Verification items for the finished model (mm, model axes). Face numbers are marked on the shaded views. A direction names the side the tool comes from. Give positions to 0.01 mm unless a question says otherwise; leave off trailing zeros. Order: outer loops, then holes, each group sorted by start corner. A loop starts at its lowest first (then second) coordinate and runs counter-clockwise, first axis right, second up.
(1) Sectioned sample at A-A on y = 0. Record the cut outline in (x, z), plus the area to 3 significant figures.
(2) Sectioned sample at D-D on z = 18.75. Record the cut outline in (x, y).
(3) Sectioned sample at C-C on y = 11.75. Record the cut outline in (x, z).
(4) Mould release check, pull along Z, two halves, no side actions. Record for the marked faces 1, 2 and 3: pulls with the +Z half, pulls with the -Z half, needs draft (parallel to the pull), parting line crosses it, or undercut.
(5) Sectioned sample at B-B on x = -59. Record the cut outline in (y, z).
(6) Access from +Z, -Z, +X, -X, +Y, -Y to the whole of each face (thin tool, end or side, straight path). Record for the marked faces 4, 5 and 6.
(7) Scan lines: L1, parallel to X at y = -1.5, z = 6.25; L2, parallel to Z at x = -62, y = 7.5; L3, parallel to Z at x = -62.5, y = 5.25. Record each from-to range of solid material in increasing order.
(8) Gauge pin test, flat ends, axial feed: pin 1 (2 mm diameter, centred on y = 3.5, z = 6.5, fed in from -X); pin 2 (3 mm diameter, centred on x = -62.5, y = -1.5, fed in from +Z); pin 3 (3 mm diameter, centred on x = -55, y = 14.89, fed in from +Z); pin 4 (1.5 mm diameter, centred on y = 11, z = 17, fed in from +X). Record the tip position at first contact, or that the pin passes through.
```python
from build123d import *

# Parameters (mm, degrees)
BOSS_EXTRUDE1_DEPTH     = 20
SKETCH2_R               = 2.5
CUT_EXTRUDE1_DEPTH      = 71.632853546
BOSS_EXTRUDE4_DEPTH     = 10
CUT_EXTRUDE2_DEPTH      = 80.703956491
CUT_EXTRUDE2_DEPTH_BACK = 80.703956491
SKETCH6_W               = 5.08
SKETCH6_H               = 17.7
SKETCH7_R               = 0.889
CUT_EXTRUDE3_DEPTH      = 73.716888558
CUT_EXTRUDE4_DEPTH      = 73.716888558
CUT_EXTRUDE4_DEPTH_BACK = 73.716888558
SKETCH8_W               = 40
SKETCH8_H               = 4.572
SKETCH8_W_2             = 60
SKETCH8_H_2             = 5
SKETCH4_R               = 7.5
SKETCH4_R_2             = 2.5
BOSS_EXTRUDE3_DEPTH     = 3
CHAMFER1_SIZE           = 5
BOSS_EXTRUDE2_START     = 3
SKETCH3_R               = 5
SKETCH3_R_2             = 2.5
BOSS_EXTRUDE2_DEPTH     = 3
CHAMFER2_SIZE           = 3


with BuildPart() as part:
    # Sketch1 → Boss-Extrude1 (new body)
    with BuildSketch(Plane.XY):
        with BuildLine():
            Line((-60.35, 6.991244524), (-0.5, 9.987492178))
            ThreePointArc((-0.5, 9.987492178), (10, 0), (-0.5, -9.987492178))
            Line((-0.5, -9.987492178), (-60.35, -6.991244524))
            ThreePointArc((-60.35, -6.991244524), (-67, 0), (-60.35, 6.991244524))
        make_face()
    extrude(amount=BOSS_EXTRUDE1_DEPTH)

    # Sketch2 → Cut-Extrude1 (cut, through all)
    with BuildSketch(Plane.XY.offset(20)):
        with Locations((-60, 0)):
            Circle(SKETCH2_R)
        Circle(SKETCH2_R)
    extrude(amount=-CUT_EXTRUDE1_DEPTH, mode=Mode.SUBTRACT)

    # Sketch5 → Boss-Extrude4 (add)
    with BuildSketch(Plane.XY):
        with BuildLine():
            Line((-60.35, 6.991244524), (-45.63025704, 7.728153385))
            Line((-45.63025704, 7.728153385), (-50.477534128, 17.202429338))
            ThreePointArc((-50.477534128, 17.202429338), (-55.254, 19.962268451), (-59.730944827, 16.739179378))
            Line((-59.730944827, 16.739179378), (-63.60774296, 6.828153385))
            Line((-63.60774296, 6.828153385), (-64.043561758, 5.713983576))
            ThreePointArc((-64.043561758, 5.713983576), (-62.287727062, 6.615610697), (-60.35, 6.991244524))
        make_face()
    extrude(amount=BOSS_EXTRUDE4_DEPTH)

    # Sketch6 → Cut-Extrude2 (cut, two sides: drawn at the far end of the back side and taken through both)
    with BuildSketch(Plane(origin=(-63.598111022, -3.183887901, 0), x_dir=(0, 0, -1), z_dir=(0.9987492177719091, 0.05000000000000006, -2.8501484999108014e-15)).offset(-CUT_EXTRUDE2_DEPTH_BACK)):
        with Locations((-5, 18.85)):
            Rectangle(SKETCH6_W, SKETCH6_H)
    extrude(amount=CUT_EXTRUDE2_DEPTH + CUT_EXTRUDE2_DEPTH_BACK, mode=Mode.SUBTRACT)

    # Sketch7 → Cut-Extrude3 (cut, through all)
    with BuildSketch(Plane.XY.offset(20)):
        with Locations((-55, 14.888622424)):
            Circle(SKETCH7_R)
    extrude(amount=-CUT_EXTRUDE3_DEPTH, mode=Mode.SUBTRACT)

    # Sketch8 → Cut-Extrude4 (cut, two sides: drawn at the far end of the back side and taken through both)
    with BuildSketch(Plane(origin=(0, 0, 0), x_dir=(1, 0, 0), z_dir=(0, 1, 0)).offset(-CUT_EXTRUDE4_DEPTH_BACK)):
        with Locations((-10, -2.286)):
            Rectangle(SKETCH8_W, SKETCH8_H)
        with Locations((-37, -17.5)):
            Rectangle(SKETCH8_W_2, SKETCH8_H_2)
    extrude(amount=CUT_EXTRUDE4_DEPTH + CUT_EXTRUDE4_DEPTH_BACK, mode=Mode.SUBTRACT)

    # Sketch4 → Boss-Extrude3 (add)
    with BuildSketch(Plane(origin=(0, 0, 4.572), x_dir=(-1, 0, 0), z_dir=(0, 0, -1))):
        with Locations(Location((0, 0, 0), (0, 0, 180))):
            Circle(SKETCH4_R)
        with Locations(Location((0, 0, 0), (0, 0, 180))):
            Circle(SKETCH4_R_2, mode=Mode.SUBTRACT)
    extrude(amount=BOSS_EXTRUDE3_DEPTH)

    # Chamfer1
    # the kernel refuses this chamfer: 5 mm, written as the material it adds along each edge
    with BuildSketch(Plane(origin=(-30, -21.369059903, 4.572), x_dir=(-0.027495876610586317, 0, -0.9996219169112968), z_dir=(0, 1, 0))) as chamfer1_piece_1_section:
        Polygon((CHAMFER1_SIZE * 0.999621916911, -CHAMFER1_SIZE * 0.0274958766106), (-CHAMFER1_SIZE * 0.0274958766106, -CHAMFER1_SIZE * 0.999621916911), (0, 0), align=None)
    chamfer1_piece_1 = extrude(amount=42.738119807, mode=Mode.PRIVATE)
    chamfer1_piece_1 = split(chamfer1_piece_1, bisect_by=Plane(origin=(-28.745975843, 8.573424695, 2.975382292), z_dir=(0.050000000000000065, -0.998749217771909, 0)), keep=Keep.TOP, mode=Mode.PRIVATE)
    chamfer1_piece_1 = split(chamfer1_piece_1, bisect_by=Plane(origin=(-28.316767762, 0, 0), z_dir=(0, 0, 1)), keep=Keep.TOP, mode=Mode.PRIVATE)
    chamfer1_piece_1 = split(chamfer1_piece_1, bisect_by=Plane(origin=(-28.745975843, -8.573424695, 2.975382292), z_dir=(0.05000000000000006, 0.998749217771909, 0)), keep=Keep.TOP, mode=Mode.PRIVATE)
    add(chamfer1_piece_1)

    # Sketch3 → Boss-Extrude2 (add)
    with BuildSketch(Plane.XY.offset(15).offset(BOSS_EXTRUDE2_START)):
        with Locations(Location((-60, 0, 0), (0, 0, 180))):
            Circle(SKETCH3_R)
        with Locations((-60, 0)):
            Circle(SKETCH3_R_2, mode=Mode.SUBTRACT)
    extrude(amount=-BOSS_EXTRUDE2_DEPTH)

    # Chamfer2
    chamfer2_edges = [part.edges().sort_by_distance(p)[0] for p in [
        (-7, 0, 20),
    ]]
    chamfer(chamfer2_edges, length=CHAMFER2_SIZE)


solid = part.part
```
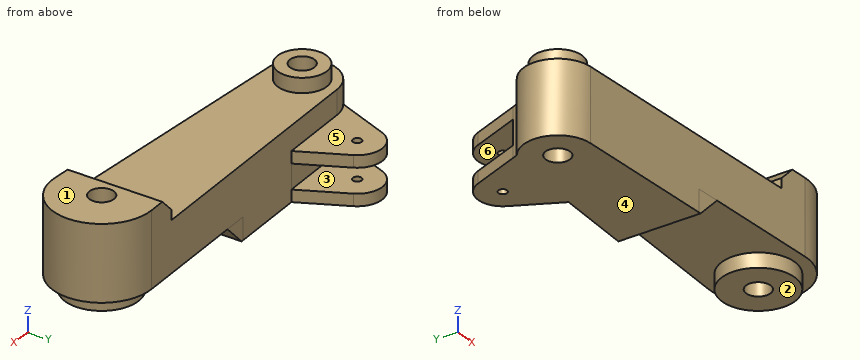
Ans:
1. outline: (-67, 0) - (-62.5, 0) - (-62.5, 18) - (-65, 18) - (-65, 15) - (-67, 15) - close; (-57.5, 0) - (-29.57, 0) - (-25, 4.57) - (-7.5, 4.57) - (-7.5, 1.57) - (-2.5, 1.57) - (-2.5, 20) - (-4, 20) - (-7, 17) - (-7, 15) - (-55, 15) - (-55, 18) - (-57.5, 18) - close; (2.5, 1.57) - (7.5, 1.57) - (7.5, 4.57) - (10, 4.57) - (10, 20) - (2.5, 20) - close
1. area: 958 mm2
2. outline: (-5.25, -9.75) - (-0.5, -9.99) arc R10 ccw (long way) to (-0.5, 9.99) - (-5.25, 9.75) - close; hole circle Ø5 at (0, 0)
3. outline: (-61.68, 0) - (-47.69, 0) - (-47.69, 2.46) - (-61.68, 2.46) - close; (-61.68, 7.54) - (-47.69, 7.54) - (-47.69, 10) - (-61.68, 10) - close
4. face 1: pulls with the +Z half
4. face 2: pulls with the -Z half
4. face 3: undercut
5. outline: (-7.06, 0) - (-2.29, 0) - (-2.29, 18) - (-4.9, 18) - (-4.9, 15) - (-7.06, 15) - close; (2.29, 0) - (18.02, 0) - (18.02, 2.46) - (7.06, 2.46) - (7.06, 7.54) - (18.02, 7.54) - (18.02, 10) - (7.06, 10) - (7.06, 15) - (4.9, 15) - (4.9, 18) - (2.29, 18) - close
6. face 4: -Z, +X, -X, +Y, -Y
6. face 5: +Z, -X, +Y
6. face 6: -X, +Y
7. L1: x = -66.84 to -62, -58 to -2, 2 to 9.89
7. L2: z = 0 to 2.46, 7.54 to 10
7. L3: z = 0 to 15
8. pin 1: stops at x = -66.54
8. pin 2: stops at z = 18
8. pin 3: stops at z = 10
8. pin 4: passes through
